Design review of the part built by this model. Coordinates are the model's own, in mm. Face numbers are marked on the shaded views. A direction names the side the tool comes from. Coordinates: 2 decimals unless noted, no trailing zeros. Write each loop counter-clockwise with the first axis right and the second up, starting at its lowest first coordinate (ties: lowest second). Pieces come first, ordered by that corner, then holes. Notation, with made-up numbers: M -12.75,86.5 L 41.25,86.5 A21 ccw 41.25,120.5 Z; hole C 85.5,5 d7. An arc over 180 degrees is marked long. Write item = value, one per line.
```python
from build123d import *

# Parameters (mm, degrees)
F0_W     = 5
F0_H     = 7.5
F0_W_2   = 7.5
F0_H_2   = 5
F1_DEPTH = 5
F2_DEPTH = 2
F3_R     = 5


with BuildPart() as f1:
    # F0 (on Top) → F1 (new body)
    with BuildSketch(Plane.XY):
        with BuildLine():
            Line((2.5, 5.4543560573), (2.5, 50))
            Line((2.5, 50), (-2.5, 50))
            Line((-2.5, 50), (-2.5, 5.4543560573))
            ThreePointArc((-2.5, 5.4543560573), (0, 6), (2.5, 5.4543560573))
        make_face()
        with BuildLine():
            ThreePointArc((5.4543560573, 2.5), (4.2426406871, 4.2426406871), (2.5, 5.4543560573))
            Line((2.5, 5.4543560573), (2.5, 2.829016319))
            Line((2.5, 2.829016319), (3.0698729811, 2.5))
            Line((3.0698729811, 2.5), (5.4543560573, 2.5))
        make_face()
        with BuildLine():
            Line((2.5, 2.829016319), (2.5, 5.4543560573))
            ThreePointArc((2.5, 5.4543560573), (0, 6), (-2.5, 5.4543560573))
            Line((-2.5, 5.4543560573), (-2.5, 2.829016319))
            Line((-2.5, 2.829016319), (0, 4.272391992))
            Line((0, 4.272391992), (2.5, 2.829016319))
        make_face()
        with BuildLine():
            Line((-2.5, 2.829016319), (-2.5, 5.4543560573))
            ThreePointArc((-2.5, 5.4543560573), (-4.2426406871, 4.2426406871), (-5.4543560573, 2.5))
            Line((-5.4543560573, 2.5), (-3.0698729811, 2.5))
            Line((-3.0698729811, 2.5), (-2.5, 2.829016319))
        make_face()
        with BuildLine():
            ThreePointArc((6, 0), (5.8620020617, 1.2794263668), (5.4543560573, 2.5))
            Line((5.4543560573, 2.5), (3.0698729811, 2.5))
            Line((3.0698729811, 2.5), (3.7, 2.136195996))
            Line((3.7, 2.136195996), (3.7, -2.136195996))
            Line((3.7, -2.136195996), (3.0698729811, -2.5))
            Line((3.0698729811, -2.5), (5.4543560573, -2.5))
            ThreePointArc((5.4543560573, -2.5), (5.8620020617, -1.2794263668), (6, 0))
        make_face()
        with BuildLine():
            Line((37.5, 2.5), (5.4543560573, 2.5))
            ThreePointArc((5.4543560573, 2.5), (5.8620020617, 1.2794263668), (6, 0))
            ThreePointArc((6, 0), (5.8620020617, -1.2794263668), (5.4543560573, -2.5))
            Line((5.4543560573, -2.5), (37.5, -2.5))
            Line((37.5, -2.5), (37.5, -2.4188727583))
            Line((37.5, -2.4188727583), (37.5, 2.5))
        make_face()
        with BuildLine():
            ThreePointArc((-5.4543560573, -2.5), (-6, 0), (-5.4543560573, 2.5))
            Line((-5.4543560573, 2.5), (-50, 2.5))
            Line((-50, 2.5), (-50, -2.5))
            Line((-50, -2.5), (-5.4543560573, -2.5))
        make_face()
        with BuildLine():
            Line((-3.0698729811, 2.5), (-5.4543560573, 2.5))
            ThreePointArc((-5.4543560573, 2.5), (-6, 0), (-5.4543560573, -2.5))
            Line((-5.4543560573, -2.5), (-3.0698729811, -2.5))
            Line((-3.0698729811, -2.5), (-3.7, -2.136195996))
            Line((-3.7, -2.136195996), (-3.7, 2.136195996))
            Line((-3.7, 2.136195996), (-3.0698729811, 2.5))
        make_face()
        with Locations((40, 6.25)):
            Rectangle(F0_W, F0_H)
        Polygon((42.5, 2.5), (37.5, 2.5), (37.5, -2.4188727583), (37.5, -2.5), (42.5, -2.5), align=None)
        Polygon((38.6080273271, -2.4188727583), (37.5, -2.4188727583), (39.1182749787, 0.0960717336), (37.6035439795, 2.4583689155), (38.7446626815, 2.4583689155), (39.7950469684, 0.7034585824), (40.8262169086, 2.4583689155), (41.9395815542, 2.4583689155), (40.4088385995, 0.0394961571), (42.0570025619, -2.4188727583), (40.8763877028, -2.4188727583), (39.7416737831, -0.574295474), align=None, mode=Mode.SUBTRACT)
        with BuildLine():
            Line((-3.0698729811, -2.5), (-5.4543560573, -2.5))
            ThreePointArc((-5.4543560573, -2.5), (-4.2426406871, -4.2426406871), (-2.5, -5.4543560573))
            Line((-2.5, -5.4543560573), (-2.5, -2.829016319))
            Line((-2.5, -2.829016319), (-3.0698729811, -2.5))
        make_face()
        with Locations((46.25, 0)):
            Rectangle(F0_W_2, F0_H_2)
        with BuildLine():
            ThreePointArc((2.5, -5.4543560573), (4.2426406871, -4.2426406871), (5.4543560573, -2.5))
            Line((5.4543560573, -2.5), (3.0698729811, -2.5))
            Line((3.0698729811, -2.5), (2.5, -2.829016319))
            Line((2.5, -2.829016319), (2.5, -5.4543560573))
        make_face()
        with BuildLine():
            ThreePointArc((2.5, -5.4543560573), (0, -6), (-2.5, -5.4543560573))
            Line((-2.5, -5.4543560573), (-2.5, -35))
            Line((-2.5, -35), (2.5, -35))
            Line((2.5, -35), (2.5, -5.4543560573))
        make_face()
        with BuildLine():
            Line((-2.5, -2.829016319), (-2.5, -5.4543560573))
            ThreePointArc((-2.5, -5.4543560573), (0, -6), (2.5, -5.4543560573))
            Line((2.5, -5.4543560573), (2.5, -2.829016319))
            Line((2.5, -2.829016319), (0, -4.272391992))
            Line((0, -4.272391992), (-2.5, -2.829016319))
        make_face()
        with Locations((40, -6.25)):
            Rectangle(F0_W, F0_H)
        Polygon((2.5, -35), (-2.5, -35), (-2.5, -40), (-0.6391059028, -40), (-0.6391059028, -38.1043836806), (-2.2840711806, -35.0423177083), (-1.1447482639, -35.0423177083), (-0.1171875, -37.0833333333), (0.9168836806, -35.0423177083), (2.0496961806, -35.0423177083), (0.4047309028, -38.0707465278), (0.4047309028, -40), (2.5, -40), align=None)
        with Locations((-6.25, -37.5)):
            Rectangle(F0_W_2, F0_H_2)
        with Locations((6.25, -37.5)):
            Rectangle(F0_W_2, F0_H_2)
        Polygon((-0.6391059028, -40), (-2.5, -40), (-2.5, -50), (2.5, -50), (2.5, -40), (0.4047309028, -40), align=None)
    extrude(amount=F1_DEPTH)

    # F0 (on Top) → F2 (join)
    with BuildSketch(Plane.XY):
        Polygon((2.5, 2.5980762114), (2.5, 2.829016319), (0, 4.272391992), (-2.5, 2.829016319), (-2.5, 2.5980762114), (0, 4.0414518843), align=None)
        Polygon((-2.6698729811, 2.5), (-3.0698729811, 2.5), (-3.7, 2.136195996), (-3.7, -2.136195996), (-3.0698729811, -2.5), (-2.6698729811, -2.5), (-3.5, -2.0207259422), (-3.5, 2.0207259422), align=None)
        Polygon((-2.5, 2.5980762114), (-2.5, 2.829016319), (-3.0698729811, 2.5), (-2.6698729811, 2.5), align=None)
        Polygon((-2.6698729811, -2.5), (-3.0698729811, -2.5), (-2.5, -2.829016319), (-2.5, -2.5980762114), align=None)
        Polygon((-2.5, -2.5980762114), (-2.5, -2.829016319), (0, -4.272391992), (2.5, -2.829016319), (2.5, -2.5980762114), (0, -4.0414518843), align=None)
        Polygon((2.5, -2.829016319), (3.0698729811, -2.5), (2.6698729811, -2.5), (2.5, -2.5980762114), align=None)
        Polygon((3.7, 2.136195996), (3.0698729811, 2.5), (2.6698729811, 2.5), (3.5, 2.0207259422), (3.5, -2.0207259422), (2.6698729811, -2.5), (3.0698729811, -2.5), (3.7, -2.136195996), align=None)
        Polygon((3.0698729811, 2.5), (2.5, 2.829016319), (2.5, 2.5980762114), (2.6698729811, 2.5), align=None)
    extrude(amount=F2_DEPTH)

    # F3
    f3_edges = [f1.edges().sort_by_distance(p)[0] for p in [
        (37.5, -2.5, 2.5),
        (-2.5, -40, 2.5),
        (-2.5, -35, 2.5),
        (37.5, 2.5, 2.5),
        (42.5, 2.5, 2.5),
        (2.5, -35, 2.5),
        (2.5, -40, 2.5),
        (42.5, -2.5, 2.5),
    ]]
    fillet(f3_edges, radius=F3_R)


solid = f1.part
```
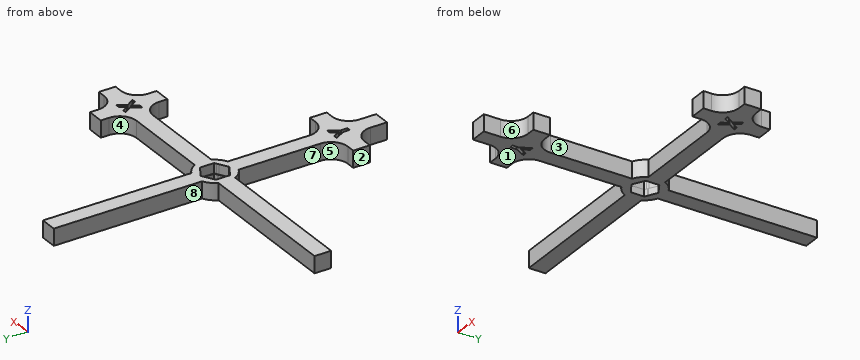
Q1. Machinability: for the marked faces 1, 2, 3, 4 and 5, which of the approach directions +Z, -Z, +X, -X, +Y, -Y give a long, thin tool a straight path to every point of the face, cutting with its end or side? Answer none if there is none.
Check result:
face_1 = -Z, +X, -X, +Y, -Y
face_2 = +Z, -Z, -X, -Y
face_3 = +Z, -Z
face_4 = +Z, -Z, +Y
face_5 = +Z, -Z, -X
Q2. For P1, Ø2.5, axis at x = 40, z = 3.5, coming from the +Y side; P2, Ø1.5, axis at y = -47.5, z = 2, coming from the +X side; P3, Ø4, axis at x = 3, y = -12, coming from the -Z side; P4, Ø0.8, axis at x = 8.5, z = 3.5, coming from the -Y side, all flat-tipped, find the tip position at first contact; note any pin that passes through.
Check result:
P1 = 10
P2 = 2.5
P3 = 0
P4 = -40
Q3. Wall thickness on line 1 (X direction, y = -7, z = 2.85); line 2 (Y direction, x = -9, z = 2.8); line 3 (X direction, y = 0.5, z = 1.75): over which ranges is each line inside the solid? List them lowest first.
Check result:
line_1 = -2.5 to 2.5, 37.47 to 42.53
line_2 = -40 to -35, -2.5 to 2.5
line_3 = -50 to -3.5, 3.5 to 38.86, 40.7 to 50
Q4. Consider section B-B, the plane z = 3.6. State how many separate pieces and enclosed holes the cut face has, and give its area (3 significant figures).
Check result:
separate_pieces = 1
enclosed_holes = 3
area = 1,120 mm²
Q5. Consider section A-A, the plane y = 39.5. State the section outline as (x, z) points.
Check result:
outline = M -2.5,0 L 2.5,0 L 2.5,5 L -2.5,5 Z
Q6. The part is to be moulded in two halves that separate along Y. For the marked faces 6, 7 and 8, say which applies: +Y half, -Y half, draft (parallel to the pull), parting line (faces both ways), or undercut.
Check result:
face_6 = -Y half
face_7 = undercut
face_8 = draft
